Geometry check sheet. Reference: the model listing, model coordinates, mm. Coordinates: 2 decimals unless noted, no trailing zeros. Order: outer loops, then holes, each group sorted by start corner. A loop starts at its lowest first (then second) coordinate and runs counter-clockwise, first axis right, second up. Notation, with made-up numbers: (-4, 17.5) - (24, 17.5) arc R23 ccw to (24, 46.5) - close; hole circle Ø10 at (8.5, 30). An arc over 180 degrees is marked (long way). One line per item, written item: value. Start each with the question number.
```python
from build123d import *

# Parameters (mm, degrees)
SKETCH1_W          = 152.4
SKETCH1_H          = 44.45
BASE_FLANGE1_DEPTH = 2.65684
CUT_EXTRUDE3_DEPTH = 159.772230881


# Sheet-metal steps are written as plain solids
with BuildPart() as part:
    # Sketch1 → Base-Flange1 (new body)
    with BuildSketch(Plane(origin=(0, 0, 0), x_dir=(1, 0, 0), z_dir=(0, 1, 0))):
        with Locations((76.2, 22.225)):
            Rectangle(SKETCH1_W, SKETCH1_H)
    extrude(amount=-BASE_FLANGE1_DEPTH)

    # Sketch10 → Cut-Extrude3 (cut, through all)
    with BuildSketch(Plane.XZ.offset(2.65684)):
        with BuildLine():
            Line((25.796875, -29.21), (31.353125, -29.21))
            ThreePointArc((31.353125, -29.21), (37.703125, -22.86), (31.353125, -16.51))
            Line((31.353125, -16.51), (25.796875, -16.51))
            ThreePointArc((25.796875, -16.51), (19.446875, -22.86), (25.796875, -29.21))
        make_face()
        with BuildLine():
            Line((121.046875, -29.21), (126.603125, -29.21))
            ThreePointArc((126.603125, -29.21), (132.953125, -22.86), (126.603125, -16.51))
            Line((126.603125, -16.51), (121.046875, -16.51))
            ThreePointArc((121.046875, -16.51), (114.696875, -22.86), (121.046875, -29.21))
        make_face()
    extrude(amount=-CUT_EXTRUDE3_DEPTH, mode=Mode.SUBTRACT)


solid = part.part
```
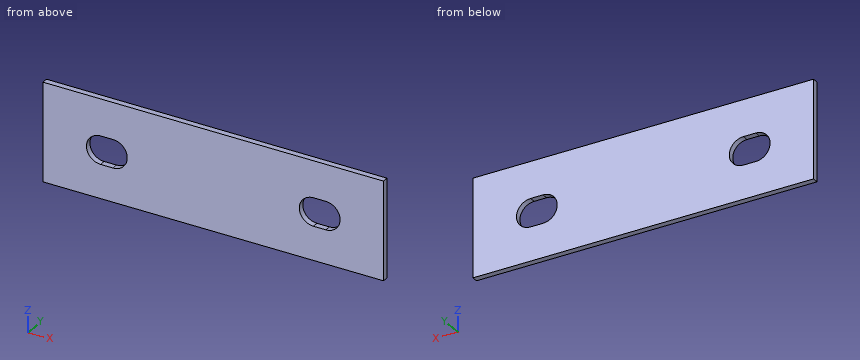
Q1. Cross-section at C-C, the plane y = -1.45. Enter the section's corners in (x, z), and give its area (3 significant figures).
Q2. Cross-section at A-A, the plane x = 27.5. Enter the section's corners in (y, z).
Q3. Cross-section at B-B, the plane z = -22.86. Enter the section's corners in (x, y), and give its area (3 significant figures).
Q4. Material ranges on probe 1 along X at (y, z) = (-2.45, -18.5); probe 2 along X at (y, z) = (-0.55, -21); probe 3 along Z at (x, y) = (32.5, -0.15), recorded low to high.
Check result:
1. outline: (0, -44.45) - (152.4, -44.45) - (152.4, 0) - (0, 0) - close; hole (25.8, -29.21) - (31.35, -29.21) arc R6.35 ccw to (31.35, -16.51) - (25.8, -16.51) arc R6.35 ccw to start; hole (121.05, -29.21) - (126.6, -29.21) arc R6.35 ccw to (126.6, -16.51) - (121.05, -16.51) arc R6.35 ccw to start
1. area: 6,380 mm2
2. outline: (-2.66, -44.45) - (0, -44.45) - (0, -29.21) - (-2.66, -29.21) - close; (-2.66, -16.51) - (0, -16.51) - (0, 0) - (-2.66, 0) - close
3. outline: (0, -2.66) - (19.45, -2.66) - (19.45, 0) - (0, 0) - close; (37.7, -2.66) - (114.7, -2.66) - (114.7, 0) - (37.7, 0) - close; (132.95, -2.66) - (152.4, -2.66) - (152.4, 0) - (132.95, 0) - close
3. area: 308 mm2
4. probe 1: x = 0 to 21.18, 35.97 to 116.43, 131.22 to 152.4
4. probe 2: x = 0 to 19.73, 37.42 to 114.98, 132.67 to 152.4
4. probe 3: z = -44.45 to -29.11, -16.61 to 0
